Can you work these out from the model? Positions are in its coordinate system, mm. Face numbers are marked on the shaded views. Round coordinates to 2 decimals unless told otherwise and drop trailing zeros. Loops run counter-clockwise (first coordinate to the right, second up) from the corner with the lowest first, then second, coordinate; pieces in that order, holes last.
(1) If I drill on line 1 along Y through (x, z) = (0, 1.7); line 2 along Y through (x, z) = (75, 11.5); line 3 along X through (y, z) = (4.5, 21.5), over which ranges is the centre line in solid material (lowest first)?
(2) Thinking about a two-plate mould opening in Y: for the marked faces 1, 2 and 3, which applies, released by +Y, released by -Y, zero draft, split by the parting line, or undercut?
(3) I want a section at C-C on y = 10. Write out the boundary of the cut face in (x, z).
(4) I want a section at A-A on x = 0. Write out the boundary of the cut face in (y, z).
(5) I want a section at B-B on z = 19.5. Write out the boundary of the cut face in (x, y), plus the area to 3 significant figures.
(6) I want a section at D-D on x = 79. Write out the boundary of the cut face in (y, z), plus the area to 3 significant figures.
(7) Will these pins go through, and if not, where does the flat tip stop? pin 1 Ø10 at (x, y) = (97.5, 3) entering from -Z; pin 2 Ø8 at (x, z) = (33, 10) entering from +Y; pin 3 Ø14 at (y, z) = (0.5, 16) entering from -X; pin 4 Ø5 at (y, z) = (11.5, 20) entering from -X.
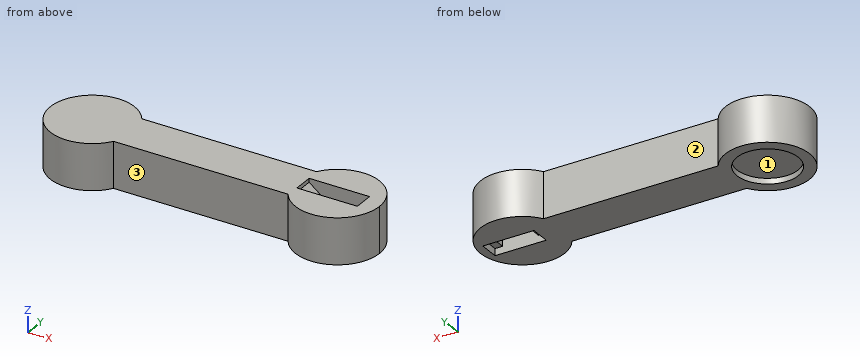
from build123d import *

# Parameters (mm, degrees)
BOSS_EXTRUDE1_DEPTH = 30
SKETCH16_W          = 33.4
SKETCH16_H          = 12.9
CUT_EXTRUDE10_DEPTH = 4.5
SKETCH17_W          = 23.45208563
SKETCH17_H          = 12.9
CUT_EXTRUDE11_DEPTH = 192.865838543
CUT_EXTRUDE13_DEPTH = 6.45
SKETCH19_R          = 20
CUT_EXTRUDE14_DEPTH = 3.65


with BuildPart() as part:
    # Sketch1 → Boss-Extrude1 (new body)
    with BuildSketch(Plane.XY):
        with BuildLine():
            ThreePointArc((187.5, 0), (167.823244805, 26.363741023), (136.951138857, 15))
            Line((136.951138857, 15), (160, 15))
            Line((160, 15), (160, -15))
            Line((160, -15), (136.951138857, -15))
            ThreePointArc((136.951138857, -15), (167.823244805, -26.363741023), (187.5, 0))
        make_face()
        with BuildLine():
            Line((160, 15), (136.951138857, 15))
            ThreePointArc((136.951138857, 15), (132.5, 0), (136.951138857, -15))
            Line((136.951138857, -15), (160, -15))
            Line((160, -15), (160, 15))
        make_face()
        with BuildLine():
            Line((136.951138857, 15), (23.048861143, 15))
            ThreePointArc((23.048861143, 15), (26.363741023, 7.823244805), (27.5, 0))
            ThreePointArc((27.5, 0), (26.363741023, -7.823244805), (23.048861143, -15))
            Line((23.048861143, -15), (136.951138857, -15))
            ThreePointArc((136.951138857, -15), (132.5, 0), (136.951138857, 15))
        make_face()
        with BuildLine():
            ThreePointArc((13.228756555, -15), (-20, 0), (13.228756555, 15))
            Line((13.228756555, 15), (23.048861143, 15))
            ThreePointArc((23.048861143, 15), (-27.5, 0), (23.048861143, -15))
            Line((23.048861143, -15), (13.228756555, -15))
        make_face()
        with BuildLine():
            Line((23.048861143, 15), (13.228756555, 15))
            ThreePointArc((13.228756555, 15), (18.228756555, 8.228756555), (20, 0))
            ThreePointArc((20, 0), (18.228756555, -8.228756555), (13.228756555, -15))
            Line((13.228756555, -15), (23.048861143, -15))
            ThreePointArc((23.048861143, -15), (26.363741023, -7.823244805), (27.5, 0))
            ThreePointArc((27.5, 0), (26.363741023, 7.823244805), (23.048861143, 15))
        make_face()
        with BuildLine():
            Line((0, -15), (0, 15))
            Line((0, 15), (13.228756555, 15))
            ThreePointArc((13.228756555, 15), (-20, 0), (13.228756555, -15))
            Line((13.228756555, -15), (0, -15))
        make_face()
        with BuildLine():
            Line((13.228756555, 15), (0, 15))
            Line((0, 15), (0, -15))
            Line((0, -15), (13.228756555, -15))
            ThreePointArc((13.228756555, -15), (18.228756555, -8.228756555), (20, 0))
            ThreePointArc((20, 0), (18.228756555, 8.228756555), (13.228756555, 15))
        make_face()
    extrude(amount=BOSS_EXTRUDE1_DEPTH)

    # Sketch16 → Cut-Extrude10 (cut)
    with BuildSketch(Plane(origin=(0, 0, 0), x_dir=(-1, 0, 0), z_dir=(0, 0, -1))):
        with Locations((-165.21934279, 0)):
            Rectangle(SKETCH16_W, SKETCH16_H)
    extrude(amount=-CUT_EXTRUDE10_DEPTH, mode=Mode.SUBTRACT)

    # Sketch17 → Cut-Extrude11 (cut, through all)
    with BuildSketch(Plane(origin=(0, 0, 0), x_dir=(-1, 0, 0), z_dir=(0, 0, -1))):
        with Locations((-165.223957185, 0)):
            Rectangle(SKETCH17_W, SKETCH17_H)
    extrude(amount=-CUT_EXTRUDE11_DEPTH, mode=Mode.SUBTRACT)

    # Sketch18 → Cut-Extrude13 (cut, symmetric)
    with BuildSketch(Plane(origin=(0, 0, 0), x_dir=(-1, 0, 0), z_dir=(0, -1, 0))):
        Polygon((-153.49791437, -15), (-153.49791437, -30), (-137.49791437, -30), (-137.49791437, -27.5), align=None)
    extrude(amount=CUT_EXTRUDE13_DEPTH, both=True, mode=Mode.SUBTRACT)

    # Sketch19 → Cut-Extrude14 (cut, symmetric)
    with BuildSketch(Plane(origin=(0, 0, 0), x_dir=(-1, 0, 0), z_dir=(0, 0, -1))):
        Circle(SKETCH19_R)
    extrude(amount=CUT_EXTRUDE14_DEPTH, both=True, mode=Mode.SUBTRACT)


solid = part.part
Filled sheet:
1. line 1: y = -27.5 to -20, 20 to 27.5
1. line 2: y = -15 to 15
1. line 3: x = -27.13 to 145.18, 176.95 to 187.13
2. face 1: undercut
2. face 2: released by +Y
2. face 3: released by -Y
3. outline: (-25.62, 0) - (-17.32, 0) - (-17.32, 3.65) - (17.32, 3.65) - (17.32, 0) - (185.62, 0) - (185.62, 30) - (-25.62, 30) - close
4. outline: (-27.5, 0) - (-20, 0) - (-20, 3.65) - (20, 3.65) - (20, 0) - (27.5, 0) - (27.5, 30) - (-27.5, 30) - close
5. outline: (23.05, -15) - (136.95, -15) arc R27.5 ccw (long way) to (136.95, 15) - (23.05, 15) arc R27.5 ccw (long way) to start; hole (147.74, -6.45) - (176.95, -6.45) - (176.95, 6.45) - (147.74, 6.45) - close
5. area: 7,610 mm2
6. outline: (-15, 0) - (15, 0) - (15, 30) - (-15, 30) - close
6. area: 900 mm2
7. pin 1: stops at z = 0
7. pin 2: stops at y = 15
7. pin 3: stops at x = -27.5
7. pin 4: stops at x = -25.99
